Geometry check sheet. Reference: drawing and pictorial views, mm from the part's lowest x, y, z. Round coordinates to 2 decimals unless told otherwise and drop trailing zeros. Order: outer loops, then holes, each group sorted by start corner. A loop starts at its lowest first (then second) coordinate and runs counter-clockwise, first axis right, second up.
Q1. Scan lines: probe 1 along Z at (x, y) = (5.5, 7) (1 decimal); probe 2 along Y at (x, z) = (1.75, 269); probe 3 along Z at (x, y) = (6, 32.5). Record each from-to range of solid material in increasing order.
Q2. Depth check by flat-ended pin: P1, Ø4, axis at x = 4, y = 54, coming from the +Z side; P2, Ø1.5, axis at x = 5, z = 200.5, coming from the -Y side; P3, Ø1.5, axis at x = 5.5, z = 285.5, coming from the +Y side. Enter the tip coordinate at first touch or a pass-through.
Q3. Cross-section at B-B on x = 9. Record the cut outline in (y, z), then the cut area to 3 significant figures.
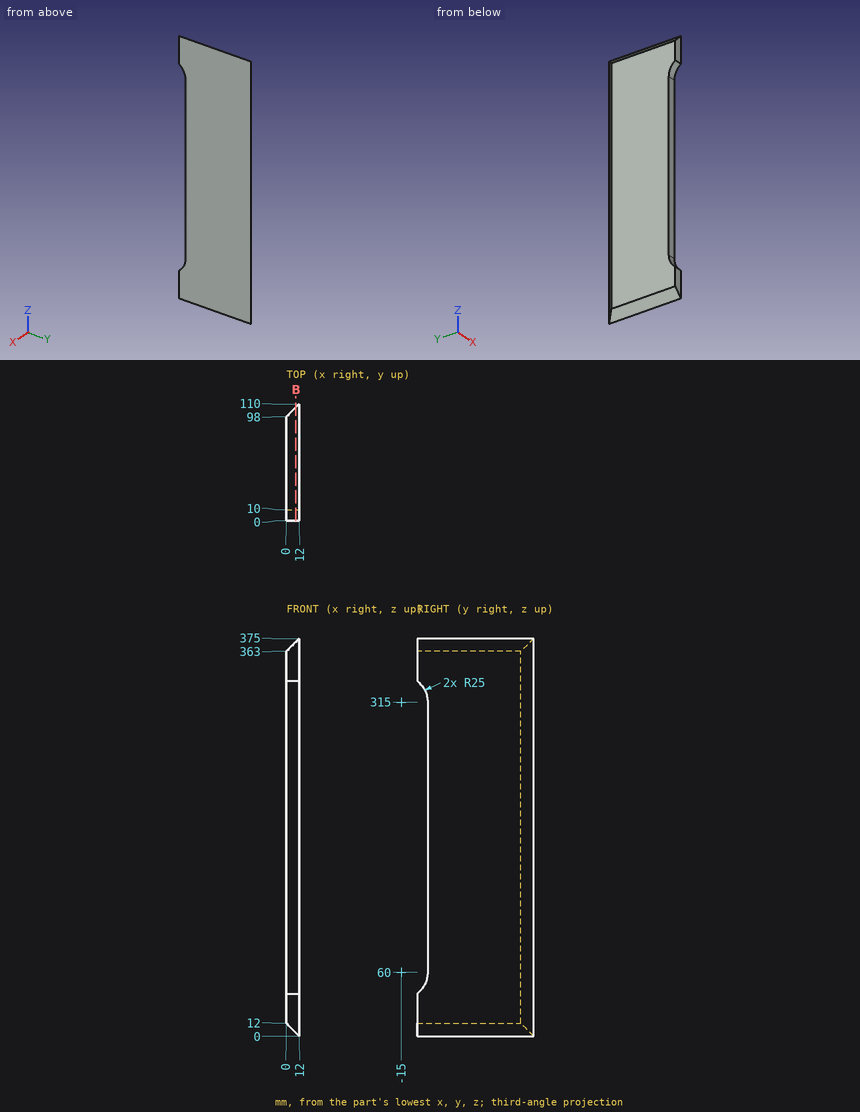
Results found:
1. probe 1: z = 6.5 to 48.1, 326.9 to 368.5
1. probe 2: y = 10 to 99.75
1. probe 3: z = 6 to 369
2. P1: stops at z = 369
2. P2: stops at y = 10
2. P3: stops at y = 104.25
3. outline: (0, 3) - (107, 3) - (107, 372) - (0, 372) - (0, 335) arc R25 cw to (10, 315) - (10, 60) arc R25 cw to (0, 40) - close
3. area: 36,700 mm2
